For this review, take the finished solid that the model builds, in its own axes (mm). Give positions to 0.01 mm unless a question says otherwise; leave off trailing zeros. Loops run counter-clockwise (first coordinate to the right, second up) from the corner with the lowest first, then second, coordinate; pieces in that order, holes last.
```python
from build123d import *

# Parameters (mm, degrees)
F0_R     = 13.5
F1_DEPTH = 5
F0_R_2   = 16.5
F2_DEPTH = 13
F3_R     = 2


# Not quite as in the source:
# - a fillet or chamfer that OpenCascade refuses, or shapes differently, is made with other operations: its cross-section is extruded or revolved along the edge and cut away or added


with BuildPart() as f1:
    # F0 (on Top) → F1 (new body)
    with BuildSketch(Plane.XY):
        Circle(F0_R)
    extrude(amount=F1_DEPTH)

    # F0 (on Top) → F2 (join)
    with BuildSketch(Plane.XY):
        Circle(F0_R_2)
        Circle(F0_R, mode=Mode.SUBTRACT)
    extrude(amount=F2_DEPTH)

    # F3
    f3_edges = [f1.edges().sort_by_distance(p)[0] for p in [
        (-16.5, 0, 13),
        (-16.5, 0, 0),
    ]]
    fillet(f3_edges, radius=F3_R)

    # F4: fillet of radius 2 on 1 edges, made by hand

    # F4_s1 → F4_t2 (revolve, cut)
    with BuildSketch(Plane.XZ):
        with BuildLine():
            ThreePointArc((14.4997999035, 13.0003463544), (13.7675927526, 12.2678330874), (13.4996, 11.2673917434))
            Line((13.4996, 11.2673917434), (13.2994634315, 11.2673917434))
            ThreePointArc((13.2994634315, 11.2673917434), (13.2998634315, 12.1336958717), (13.2998634315, 13))
            Line((13.2998634315, 13), (13.5, 13.2001365685))
            ThreePointArc((13.5, 13.2001365685), (13.9998999517, 13.2001365685), (14.3996833253, 13.1736418155))
            Line((14.3996833253, 13.1736418155), (14.4997999035, 13.0003463544))
        make_face()
    revolve(axis=Axis((0, 0, 13), (0, 0, 1)), mode=Mode.SUBTRACT)


with BuildPart() as f5_1:
    # F5: copy of F1
    add(f1.part)


with BuildPart() as f7_1:
    # F7: copy of F1
    add(f1.part.moved(Location((0, 36, 0))))


with BuildPart() as f8_1:
    # F8: copy of F1
    add(f1.part.moved(Location((36.3, 0, 0))))


with BuildPart() as f9_1:
    # F9: copy of F8_1
    add(f8_1.part.moved(Location((-0.4, 35.2, 0))))


solid = f1.part
```
Item 1: Take a section at C-C on z = 7.25. Give the boundary of the cut face in (x, y), and give its area (3 significant figures).
Answer:
outline: circle Ø33 at (0, 0); hole circle Ø27 at (0, 0)
area: 283 mm2
Item 2: The part is to be moulded in two halves that separate along Y. For faces 1 (the cylindrical face through (15.24, -6.32, 6.44)), 2 (the flat face through (0, 0, 0)), 3 (the flat face through (0, 0, 5)), say which applies: released by +Y, released by -Y, zero draft, split by the parting line, or undercut.
Answer:
face 1: split by the parting line
face 2: zero draft
face 3: undercut
Item 3: Clearance check with flat-ended pins moving along their axes: pin 1 Ø10 at (x, y) = (2, 6) entering from -Z; pin 2 Ø3 at (y, z) = (2.5, 8.5) entering from -X; pin 3 Ø3 at (x, z) = (8, 5) entering from -Y; pin 4 Ø1 at (x, z) = (5.5, 4) entering from +Y. State where each tip first meets the part, or that it passes through.
Answer:
pin 1: stops at z = 0
pin 2: stops at x = -16.47
pin 3: stops at y = -15.17
pin 4: stops at y = 15.72
Item 4: For L1, parallel to Y at x = 0, z = 7.25; L2, parallel to Z at x = 2.5, y = 4; L3, parallel to X at y = 5, z = 6, list the stretches that pass through material, from the lowest coordinate up.
Answer:
L1: y = -16.5 to -13.5, 13.5 to 16.5
L2: z = 0 to 5
L3: x = -15.72 to -12.54, 12.54 to 15.72
